Read the model definition and answer for the solid it produces. Units are mm, in the model's axes. Face numbers are marked on the shaded views. A direction names the side the tool comes from. Give positions to 0.01 mm unless a question says otherwise; leave off trailing zeros. Order: outer loops, then holes, each group sorted by start corner. A loop starts at its lowest first (then second) coordinate and runs counter-clockwise, first axis right, second up. Notation, with made-up numbers: (61, -16) - (116, -16) arc R11 cw to (116, 0) - close; hole circle Ø7 at (82, 69.5). An arc over 180 degrees is marked (long way). Write each question's results on one line, items separated by ' | '. Start each with the question number.
Q1. A tool of negligible diameter and unlimited length cuts with its end or side. For the marked faces 4 and 5, from which of +Z, -Z, +X, -X, +Y, -Y can it reach the whole face along a straight path? Write none if from no direction.
Q2. Find section A-A on y = -4.5. Give the vertices of the cut face in (x, z) (3 decimals).
Q3. For a pull along X with two mould halves and no side action, classify the marked faces 1, 2 and 3 as +X half, -X half, draft (parallel to the pull), parting line (faces both ways), or undercut.
Q4. Find section B-B on x = 3.25. Give the vertices of the cut face in (y, z).
Q5. Flat-ended cylindrical pins translate along their axes: P1, Ø6, axis at x = 3, y = -10, coming from the +Z side; P2, Ø3.5, axis at x = 1.4, y = -8.61, coming from the -Z side; P3, Ø8, axis at x = 9, y = -15.5, coming from the -Z side. Find the tip coordinate at first contact, or state that the pin passes through.
Q6. Find the intervals of material crossed by line 1 along X through (y, z) = (-9, 11.25) (3 decimals); line 2 along Y through (x, z) = (0.25, 6.75); line 3 along Y through (x, z) = (4, 3.25), in increasing order. Write a range as from..to.
Q7. Find section C-C on z = 10.5. Give the vertices of the cut face in (x, y) (3 decimals).
Q8. Find section D-D on z = 4. Give the vertices of the cut face in (x, y) (1 decimal).
from build123d import *

# Parameters (mm, degrees)
SKETCH1_W               = 21.59
SKETCH1_H               = 35.56
SKETCH1_R               = 2.8575
BOSS_EXTRUDE1_DEPTH     = 12.7
SKETCH2_W               = 16.51
SKETCH2_H               = 30.48
CUT_EXTRUDE1_DEPTH      = 7.62
FILLET1_R               = 1.27
SKETCH3_W               = 0.254
SKETCH3_H               = 25.4
CUT_EXTRUDE3_DEPTH      = 1
CUT_EXTRUDE3_DEPTH_BACK = 22.59
SKETCH1_2_W             = 21.59
SKETCH1_2_H             = 35.56
SKETCH1_2_R             = 2.8575
BOSS_EXTRUDE2_DEPTH     = 5.08


with BuildPart() as part:
    # Sketch1 → Boss-Extrude1 (new body)
    with BuildSketch(Plane.XY):
        with Locations((1.27, -2.511399464)):
            Rectangle(SKETCH1_W, SKETCH1_H)
        with Locations((1.397, 5.108600536)):
            Circle(SKETCH1_R, mode=Mode.SUBTRACT)
        with Locations((1.397, -8.607399464)):
            Circle(SKETCH1_R, mode=Mode.SUBTRACT)
    extrude(amount=BOSS_EXTRUDE1_DEPTH)

    # Sketch2 → Cut-Extrude1 (cut)
    with BuildSketch(Plane.XY.offset(12.7)):
        with Locations((1.27, -2.511399464)):
            Rectangle(SKETCH2_W, SKETCH2_H)
    extrude(amount=-CUT_EXTRUDE1_DEPTH, mode=Mode.SUBTRACT)

    # Fillet1
    fillet1_edges = [part.edges().sort_by_distance(p)[0] for p in [
        (-6.985, -17.751399464, 8.89),
        (-6.985, 12.728600536, 8.89),
        (9.525, 12.728600536, 8.89),
        (9.525, -17.751399464, 8.89),
        (-9.525, 15.268600536, 6.35),
        (12.065, 15.268600536, 6.35),
        (12.065, -20.291399464, 6.35),
        (-9.525, -20.291399464, 6.35),
    ]]
    fillet(fillet1_edges, radius=FILLET1_R)

    # Sketch3 → Cut-Extrude3 (cut, two sides)
    with BuildSketch(Plane(origin=(12.065, 0, 0), x_dir=(0, 0, -1), z_dir=(1, 0, 0))) as cut_extrude3_sk:
        with Locations((-8.255, -0.606399464)):
            Rectangle(SKETCH3_W, SKETCH3_H)
    extrude(amount=CUT_EXTRUDE3_DEPTH, mode=Mode.SUBTRACT)
    extrude(cut_extrude3_sk.sketch, amount=-CUT_EXTRUDE3_DEPTH_BACK, mode=Mode.SUBTRACT)

    # Sketch1<2> → Boss-Extrude2 (add)
    with BuildSketch(Plane.XY):
        with Locations((1.27, -2.511399464)):
            Rectangle(SKETCH1_2_W, SKETCH1_2_H)
        with Locations((1.397, 5.108600536)):
            Circle(SKETCH1_2_R, mode=Mode.SUBTRACT)
        with Locations((1.397, -8.607399464)):
            Circle(SKETCH1_2_R, mode=Mode.SUBTRACT)
    extrude(amount=BOSS_EXTRUDE2_DEPTH)


solid = part.part
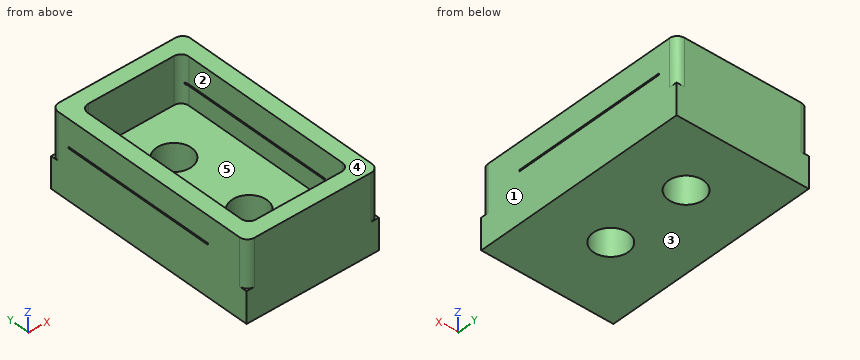
Working result:
1) face 4: +Z, +X, -X, +Y, -Y | face 5: +Z
2) outline: (-9.525, 0) - (12.065, 0) - (12.065, 8.128) - (9.525, 8.128) - (9.525, 5.08) - (-6.985, 5.08) - (-6.985, 8.128) - (-9.525, 8.128) - close; (-9.525, 8.382) - (-6.985, 8.382) - (-6.985, 12.7) - (-9.525, 12.7) - close; (9.525, 8.382) - (12.065, 8.382) - (12.065, 12.7) - (9.525, 12.7) - close
3) face 1: +X half | face 2: undercut | face 3: draft
4) outline: (-20.29, 0) - (-10.78, 0) - (-10.78, 5.08) - (-17.75, 5.08) - (-17.75, 12.7) - (-20.29, 12.7) - close; (-6.43, 0) - (2.93, 0) - (2.93, 5.08) - (-6.43, 5.08) - close; (7.28, 0) - (15.27, 0) - (15.27, 12.7) - (12.73, 12.7) - (12.73, 5.08) - (7.28, 5.08) - close
5) P1: z = 5.08 | P2: through | P3: z = 0
6) line 1: -9.525..-6.985, 9.525..12.065 | line 2: -20.29..-17.75, 12.73..15.27 | line 3: -20.29..-9.79, -7.43..3.93, 6.29..15.27
7) outline: (-9.525, -19.021) arc R1.27 ccw to (-8.255, -20.291) - (10.795, -20.291) arc R1.27 ccw to (12.065, -19.021) - (12.065, 13.999) arc R1.27 ccw to (10.795, 15.269) - (-8.255, 15.269) arc R1.27 ccw to (-9.525, 13.999) - close; hole (-6.985, -16.481) arc R1.27 ccw to (-5.715, -17.751) - (8.255, -17.751) arc R1.27 ccw to (9.525, -16.481) - (9.525, 11.459) arc R1.27 ccw to (8.255, 12.729) - (-5.715, 12.729) arc R1.27 ccw to (-6.985, 11.459) - close
8) outline: (-9.5, -20.3) - (12.1, -20.3) - (12.1, 15.3) - (-9.5, 15.3) - close; hole circle Ø5.7 at (1.4, -8.6); hole circle Ø5.7 at (1.4, 5.1)
